Here's how the part is built. I have some questions about the finished solid (model axes, mm). A direction names the side the tool comes from. Round coordinates to 2 decimals unless told otherwise and drop trailing zeros. Order: outer loops, then holes, each group sorted by start corner. A loop starts at its lowest first (then second) coordinate and runs counter-clockwise, first axis right, second up.
Autodesk Inventor part; units mm, degrees
ref_plane "YZ Plane" through (0, 0, 0) normal (1, 0, 0) x (0, 1, 0)
ref_plane "XZ Plane" through (0, 0, 0) normal (0, 1, 0) x (-1, 0, 0)
ref_plane "XY Plane" through (0, 0, 0) normal (0, 0, 1) x (1, 0, 0)
sketch "スケッチ1" plane through (0, 0, 0) normal (0, 0, 1) x (1, 0, 0)
  circle A0 centre (0, 0) radius 30
  dimension "d0" = 60
extrude "押し出し1" add sketch "スケッチ1" along normal blind 2
sketch "スケッチ2" plane through (0, 0, 2) normal (0, 0, 1) x (1, 0, 0)
  circle A0 centre (0, 0) radius 8.5
  dimension "d3" = 17
extrude "押し出し2" add sketch "スケッチ2" along normal blind 20
sketch "スケッチ3" plane through (0, 0, 22) normal (0, 0, 1) x (1, 0, 0)
  point P0 (0, 0)
hole "穴1" at (0, 0, 22) direction (0, 0, -1) diameter 5 end through all
sketch "スケッチ4" plane through (0, 0, 2) normal (0, 0, 1) x (1, 0, 0)
  circle A0 centre (0, 0) radius 30
  circle A1 centre (0, 0) radius 30
  circle A2 centre (0, 0) radius 8.5
  circle A3 centre (0, 0) radius 28
  dimension "d13" = 2
extrude "押し出し3" add sketch "スケッチ4" along normal blind 7 contours A0
properties part number "wheel" material "アルミニウム 6061"
1. If we section it at C-C, the plane z = 5.5: Write out the boundary of the cut face in (x, y).
Evaluation:
outline: circle Ø60 at (0, 0); circle Ø17 at (0, 0); hole circle Ø56 at (0, 0); hole circle Ø5 at (0, 0)
2. If we mould it in two halves opening along X, with no side actions, what happens to faces 3 (the cylindrical face through (-29.97, -1.32, 4.44)), 4 (the cylindrical face through (25.865, 10.724, 5.451)), 5 (the flat face through (-25, 13, 9)), 6 (the flat face through (6, 7, 2))? For each: released by +X, released by -X, zero draft, split by the parting line, or undercut.
Evaluation:
face 3: split by the parting line
face 4: undercut
face 5: zero draft
face 6: undercut
3. If we section it at A-A, the plane y = 0: Write out the boundary of the cut face in (x, z).
Evaluation:
outline: (-30, 0) - (-2.5, 0) - (-2.5, 22) - (-8.5, 22) - (-8.5, 2) - (-28, 2) - (-28, 9) - (-30, 9) - close; (2.5, 0) - (30, 0) - (30, 9) - (28, 9) - (28, 2) - (8.5, 2) - (8.5, 22) - (2.5, 22) - close
4. If we section it at D-D, the plane x = 21: Write out the boundary of the cut face in (y, z).
Evaluation:
outline: (-21.42, 0) - (21.42, 0) - (21.42, 9) - (18.52, 9) - (18.52, 2) - (-18.52, 2) - (-18.52, 9) - (-21.42, 9) - close
5. I'm going to push flat-ended pins straight in: P1, Ø5, axis at y = -24, z = 5, coming from the +X side; P2, Ø1, axis at y = 16.5, z = 2.5, coming from the -X side; P3, Ø1, axis at x = -2.5, z = 19.5, coming from the -Y side. Where does each tip first touch, or does it pass through?
Evaluation:
P1: stops at x = 20.92
P2: stops at x = -25.38
P3: stops at y = -8.26
6. I need wall thicknesses on probe 1 along Y at (x, z) = (0, 4.5); probe 2 along Y at (x, z) = (0, 17); probe 3 along Z at (x, y) = (27, -7). Which ranges of each line are inside material? Lowest first, please.
Evaluation:
probe 1: y = -30 to -28, -8.5 to -2.5, 2.5 to 8.5, 28 to 30
probe 2: y = -8.5 to -2.5, 2.5 to 8.5
probe 3: z = 0 to 2
7. On a 3-axis mill with a long thin cutter (end or side, diameter ignored), from which of +Z, -Z, +X, -X, +Y, -Y can I reach the whole of each face in a straight line? I mean faces 1 (the flat face through (0, -6, 0)), 2 (the cylindrical face through (4.57, -7.167, 11.86)). Say none if no direction works.
Evaluation:
face 1: -Z, +X, -X, +Y, -Y
face 2: +Z
